```python
from build123d import *

# Parameters (mm, degrees)
SKETCH1_W                          = 95.25
SKETCH1_H                          = 95.25
BASE_EXTRUDE_DEPTH                 = 6.35
PI_SLOT_DEPTH                      = 3.175
CHAMFER1_SIZE                      = 3.81
CHAMFER2_SIZE                      = 1.905
CAMERA_START                       = 6.35
SKETCH3_W                          = 45.72
SKETCH3_H                          = 31.75
CAMERA_SLOT_DEPTH                  = 3.175
FILLET1_R                          = 1
CHAMFER3_SIZE                      = 1.905
CHAMFER3_SIZE2                     = 3.905828818
FILLET2_R                          = 7.46
F_3_16_0_1875_DIAMETER_HOLE1_D     = 4.7625
F_3_16_0_1875_DIAMETER_HOLE1_DEPTH = 9.525
F_3_16_0_1875_DIAMETER_HOLE1_TIP   = 1.430799349
F_3_5_3_5_DIAMETER_HOLE1_D         = 3.5
F_3_5_3_5_DIAMETER_HOLE1_DEPTH     = 4.064
F_3_5_3_5_DIAMETER_HOLE1_TIP       = 1.051506083


with BuildPart() as part:
    # Sketch1 → Base Extrude (new body)
    with BuildSketch(Plane(origin=(0, 0, 0), x_dir=(1, 0, 0), z_dir=(0, 1, 0))):
        Rectangle(SKETCH1_W, SKETCH1_H)
    extrude(amount=BASE_EXTRUDE_DEPTH)

    # Sketch2 → Pi Slot (add)
    with BuildSketch(Plane(origin=(0, 6.35, 0), x_dir=(1, 0, 0), z_dir=(0, 1, 0))):
        Polygon((-34.534633186, -28.575), (-42.33681664, -28.575), (-42.33681664, -6), (-47.625, -6), (-47.625, -47.625), (-34.534633186, -47.625), align=None)
        Polygon((2.325611102, -28.575), (2.325611102, -47.625), (47.625, -47.625), (47.625, -27.183287233), (44.02318336, -27.183287233), (44.02318336, -28.575), align=None)
        Polygon((-47.625, 47.625), (-47.625, 6), (-42.33681664, 6), (-42.33681664, 28.575), (44.02318336, 28.575), (44.02318336, 26.009127411), (47.625, 26.009127411), (47.625, 47.625), align=None)
    extrude(amount=PI_SLOT_DEPTH)

    # Chamfer1
    # the kernel refuses this chamfer: 3.81 mm, written as the material it takes off along each edge
    with BuildSketch(Plane(origin=(2.325611102, 9.525, 18.776887816), x_dir=(-0.027495876610586382, -0.9996219169112968, 0), z_dir=(0, 0, 1))) as chamfer1_piece_1_section:
        Polygon((CHAMFER1_SIZE * 0.999621916911, CHAMFER1_SIZE * 0.0274958766106), (-CHAMFER1_SIZE * 0.0274958766106, CHAMFER1_SIZE * 0.999621916911), (0, 0), align=None)
    chamfer1_piece_1 = extrude(amount=38.646224368, mode=Mode.PRIVATE)
    chamfer1_piece_1 = split(chamfer1_piece_1, bisect_by=Plane(origin=(3.62873216, 6.35, 38.1), z_dir=(0, 1, 0)), keep=Keep.TOP, mode=Mode.PRIVATE)
    add(chamfer1_piece_1, mode=Mode.SUBTRACT)
    with BuildSketch(Plane(origin=(-34.534633186, 9.525, 57.423112184), x_dir=(-0.9996219169112968, 0.02749587661058636, 0), z_dir=(0, 0, -1))) as chamfer1_piece_2_section:
        Polygon((CHAMFER1_SIZE * 0.999621916911, -CHAMFER1_SIZE * 0.0274958766106), (-CHAMFER1_SIZE * 0.0274958766106, -CHAMFER1_SIZE * 0.999621916911), (0, 0), align=None)
    chamfer1_piece_2 = extrude(amount=38.646224368, mode=Mode.PRIVATE)
    chamfer1_piece_2 = split(chamfer1_piece_2, bisect_by=Plane(origin=(-35.837754245, 6.35, 38.1), z_dir=(0, 1, 0)), keep=Keep.TOP, mode=Mode.PRIVATE)
    add(chamfer1_piece_2, mode=Mode.SUBTRACT)
    with BuildSketch(Plane(origin=(-32.538704456, 9.525, 6), x_dir=(0, 0.027495876610586386, 0.9996219169112968), z_dir=(-1, 0, 0))) as chamfer1_piece_3_section:
        Polygon((CHAMFER1_SIZE * 0.999621916911, -CHAMFER1_SIZE * 0.0274958766106), (-CHAMFER1_SIZE * 0.0274958766106, -CHAMFER1_SIZE * 0.999621916911), (0, 0), align=None)
    chamfer1_piece_3 = extrude(amount=24.884407728, mode=Mode.PRIVATE)
    chamfer1_piece_3 = split(chamfer1_piece_3, bisect_by=Plane(origin=(-44.98090832, 6.35, 7.303121058), z_dir=(0, 1, 0)), keep=Keep.TOP, mode=Mode.PRIVATE)
    add(chamfer1_piece_3, mode=Mode.SUBTRACT)
    with BuildSketch(Plane(origin=(-57.423112184, 9.525, -6), x_dir=(0, -0.9996219169112968, 0.027495876610586382), z_dir=(1, 0, 0))) as chamfer1_piece_4_section:
        Polygon((CHAMFER1_SIZE * 0.999621916911, CHAMFER1_SIZE * 0.0274958766106), (-CHAMFER1_SIZE * 0.0274958766106, CHAMFER1_SIZE * 0.999621916911), (0, 0), align=None)
    chamfer1_piece_4 = extrude(amount=24.884407728, mode=Mode.PRIVATE)
    chamfer1_piece_4 = split(chamfer1_piece_4, bisect_by=Plane(origin=(-44.98090832, 6.35, -7.303121058), z_dir=(0, 1, 0)), keep=Keep.TOP, mode=Mode.PRIVATE)
    add(chamfer1_piece_4, mode=Mode.SUBTRACT)

    # Chamfer2
    chamfer2_edges = [part.edges().sort_by_distance(p)[0] for p in [
        (-42.984816593, 9.525, 47.625),
        (47.625, 9.525, 37.404143616),
        (47.625, 9.525, -36.817063706),
        (0, 9.525, -47.625),
        (-47.625, 9.525, -28.7175),
        (26.880305551, 9.525, 47.625),
        (-47.625, 9.525, 28.7175),
    ]]
    chamfer(chamfer2_edges, length=CHAMFER2_SIZE)

    # Sketch3 → Camera Slot (add)
    with BuildSketch(Plane(origin=(0, 0, 0), x_dir=(1, 0, 0), z_dir=(0, 1, 0)).offset(CAMERA_START)):
        with Locations((-70.485, 0)):
            Rectangle(SKETCH3_W, SKETCH3_H)
        with BuildLine():
            Line((-89.535, 11.684), (-57.785, 11.684))
            ThreePointArc((-57.785, 11.684), (-56.642, 10.541), (-57.785, 9.398))
            Line((-57.785, 9.398), (-89.535, 9.398))
            ThreePointArc((-89.535, 9.398), (-90.678, 10.541), (-89.535, 11.684))
        make_face(mode=Mode.SUBTRACT)
        with BuildLine():
            Line((-89.535, -11.684), (-57.785, -11.684))
            ThreePointArc((-57.785, -11.684), (-56.642, -10.541), (-57.785, -9.398))
            Line((-57.785, -9.398), (-89.535, -9.398))
            ThreePointArc((-89.535, -9.398), (-90.678, -10.541), (-89.535, -11.684))
        make_face(mode=Mode.SUBTRACT)
    extrude(amount=-CAMERA_SLOT_DEPTH)

    # Fillet1
    fillet1_edges = [part.edges().sort_by_distance(p)[0] for p in [
        (-93.345, 4.7625, -15.875),
        (-93.345, 4.7625, 15.875),
    ]]
    fillet(fillet1_edges, radius=FILLET1_R)

    # Chamfer3
    chamfer3_edges = [part.edges().sort_by_distance(p)[0] for p in [
        (-47.625, 3.175, 0),
    ]]
    chamfer3_side = [part.faces().sort_by_distance(p)[0] for p in [
        (-47.625, 3.81, 46.669456861),
    ]]
    chamfer(chamfer3_edges, length=CHAMFER3_SIZE, length2=CHAMFER3_SIZE2, reference=chamfer3_side[0])

    # Fillet2
    # the kernel refuses this fillet: 7.46 mm, written as the material it adds along each edge
    with BuildSketch(Plane(origin=(-47.625, 6.35, -15.875), x_dir=(-1, 0, 0), z_dir=(0, 0, 1))) as fillet2_piece_1_section:
        with BuildLine():
            CenterArc((4.163592199, -7.46), FILLET2_R, 90, 33.926040017)
            Line((0, -1.27), (0, 0))
            Line((0, 0), (4.163592199, 0))
        make_face()
    fillet2_piece_1 = extrude(amount=19.648980498, mode=Mode.PRIVATE)
    fillet2_piece_1 = split(fillet2_piece_1, bisect_by=Plane(origin=(-49.607751226, 8.8151447, -9.1001447), z_dir=(0, -0.7071067811868302, -0.7071067811862648)), keep=Keep.TOP, mode=Mode.PRIVATE)
    add(fillet2_piece_1)
    with BuildSketch(Plane(origin=(-47.625, 6.35, -3.773980498), x_dir=(-1, 0, 0), z_dir=(0, 0, 1))) as fillet2_piece_2_section:
        with BuildLine():
            CenterArc((4.163592199, -7.46), FILLET2_R, 90, 33.926040017)
            Line((0, -1.27), (0, 0))
            Line((0, 0), (4.163592199, 0))
        make_face()
    fillet2_piece_2 = extrude(amount=19.648980498, mode=Mode.PRIVATE)
    fillet2_piece_2 = split(fillet2_piece_2, bisect_by=Plane(origin=(-49.607751226, 8.8151447, 9.1001447), z_dir=(0, -0.7071067811862648, 0.7071067811868302)), keep=Keep.TOP, mode=Mode.PRIVATE)
    add(fillet2_piece_2)

    # 3/16 (0.1875) Diameter Hole1
    with Locations(Plane(origin=(0, 9.525, 0), x_dir=(1, 0, 0), z_dir=(0, 1, 0))):
        with Locations((-42.207203769, 42.207203769), (42.207203769, 42.207203769), (42.207203769, -42.207203769), (-42.207203769, -42.207203769)):
            Hole(F_3_16_0_1875_DIAMETER_HOLE1_D / 2, depth=F_3_16_0_1875_DIAMETER_HOLE1_DEPTH)
            with Locations((0, 0, -(F_3_16_0_1875_DIAMETER_HOLE1_DEPTH + F_3_16_0_1875_DIAMETER_HOLE1_TIP / 2))):  # 118° drill point
                Cone(0, F_3_16_0_1875_DIAMETER_HOLE1_D / 2, F_3_16_0_1875_DIAMETER_HOLE1_TIP, mode=Mode.SUBTRACT)

    # Ø3.5 (3.5) Diameter Hole1
    with Locations(Plane(origin=(0, 6.35, 0), x_dir=(1, 0, 0), z_dir=(0, 1, 0))):
        with Locations((-38.178407454, 24.41003259), (19.821592546, 24.41003259), (19.821592546, -24.589967454), (-38.178407454, -24.589967454)):
            Hole(F_3_5_3_5_DIAMETER_HOLE1_D / 2, depth=F_3_5_3_5_DIAMETER_HOLE1_DEPTH)
            with Locations((0, 0, -(F_3_5_3_5_DIAMETER_HOLE1_DEPTH + F_3_5_3_5_DIAMETER_HOLE1_TIP / 2))):  # 118° drill point
                Cone(0, F_3_5_3_5_DIAMETER_HOLE1_D / 2, F_3_5_3_5_DIAMETER_HOLE1_TIP, mode=Mode.SUBTRACT)


solid = part.part
```
Verification items for the finished model (mm, model axes). A direction names the side the tool comes from. Give positions to 0.01 mm unless a question says otherwise; leave off trailing zeros. Order: outer loops, then holes, each group sorted by start corner. A loop starts at its lowest first (then second) coordinate and runs counter-clockwise, first axis right, second up. Notation, with made-up numbers: (61.5, 12) - (87.5, 12) arc R18 ccw to (87.5, 33) - close; hole circle Ø6 at (-31, -3). An arc over 180 degrees is marked (long way). Answer as CSV lines item,"result". Start each with the question number.
Item 1: Gauge pin test, flat ends, axial feed: pin 1 (5 mm diameter, centred on x = -79.5, y = 3.5, fed in from -Z) (3 decimals); pin 2 (1 mm diameter, centred on x = -17, y = 8, fed in from +Z) (3 decimals); pin 3 (0.7 mm diameter, centred on y = 8.5, z = 27.5, fed in from -X) (3 decimals). Record the tip position at first contact, or that the pin passes through.
Item 2: Section check D-D, the plane x = 36. Record the boundary of the cut face in (y, z) (3 decimals).
Item 3: Mould release check, pull along X, two halves, no side actions. Record for faces 1 (the face through (-1, 0, -1)), 2 (the face through (-39.795, 4.29, -23.74)), 3 (the face through (-93.345, 5, 0)), 4 (the face through (-39, 8, 28.575)): released by +X, released by -X, zero draft, split by the parting line, or undercut.
Item 4: Material ranges on L1, parallel to Z at x = -80, y = 6 (3 decimals); L2, parallel to Z at x = 32, y = 6.75 (3 decimals); L3, parallel to Z at x = -57, y = 5.75 (3 decimals), recorded low to high.
Item 5: Access from +Z, -Z, +X, -X, +Y, -Y to the whole of each face (thin tool, end or side, straight path). Record for faces 5 (the face through (-45.028, 7.562, 7.847)), 6 (the face through (21.21, 4.29, -23.345)), 7 (the face through (45, 8, -26.009)).
Item 6: Section check C-C, the plane y = 4.75. State how many separate pieces and enclosed holes the cut face has, plus the area to 3 significant figures.
Item 7: Section check B-B, the plane z = 32. Record the boundary of the cut face in (x, y) (3 decimals).
Item 8: Section check A-A, the plane x = -67. Record the boundary of the cut face in (y, z) (3 decimals), plus the area to 3 significant figures.
Filled in:
1,pin 1,"z = -15.875"
1,pin 2,"z = -28.575"
1,pin 3,"x = -47.095"
2,outline,"(0, -47.625) - (7.62, -47.625) - (9.525, -45.72) - (9.525, -28.575) - (6.35, -28.575) - (6.35, 28.575) - (9.525, 28.575) - (9.525, 45.72) - (7.62, 47.625) - (0, 47.625) - close"
3,face 1,"zero draft"
3,face 2,"undercut"
3,face 3,"released by -X"
3,face 4,"undercut"
4,L1,"-15.875 to -11.684, -9.398 to 9.398, 11.684 to 15.875"
4,L2,"-47.625 to -28.575, 28.575 to 47.625"
4,L3,"-15.875 to -11.372, -9.71 to 9.71, 11.372 to 15.875"
5,face 5,"+X, -X, +Y"
5,face 6,"+Y"
5,face 7,"+X, +Y"
6,separate pieces,"1"
6,enclosed holes,"10"
6,area,"10,300 mm^2"
7,outline,"(-47.625, 0) - (47.625, 0) - (47.625, 7.62) - (45.72, 9.525) - (6.136, 9.525) - (2.961, 6.35) - (-35.17, 6.35) - (-38.345, 9.525) - (-45.72, 9.525) - (-47.625, 7.62) - close"
8,outline,"(3.175, -15.875) - (6.35, -15.875) - (6.35, -11.684) - (3.175, -11.684) - close; (3.175, -9.398) - (6.35, -9.398) - (6.35, 9.398) - (3.175, 9.398) - close; (3.175, 11.684) - (6.35, 11.684) - (6.35, 15.875) - (3.175, 15.875) - close"
8,area,"86.3 mm^2"
